For this review, take the finished solid that the model builds, in its own axes (mm). Round coordinates to 2 decimals unless told otherwise and drop trailing zeros. Write each loop counter-clockwise with the first axis right and the second up, starting at its lowest first coordinate (ties: lowest second). Pieces come first, ordered by that corner, then holes. Notation, with made-up numbers: (27, -24.75) - (74, -24.75) arc R14 cw to (74, -20.75) - close; hole circle Ø7 at (83, 89.5). An arc over 180 degrees is marked (long way). One line per item, written item: value. Start each with the question number.
Q1. Add section C-C on z = -33.5. Write out the cut boundary in (x, y), and give its area (3 significant figures).
Q2. Clearance check with flat-ended pins moving along their axes: pin 1 Ø12 at (y, z) = (2.5, -12) entering from -X; pin 2 Ø3.5 at (x, y) = (0, 28.5) entering from +Z; pin 3 Ø7 at (x, y) = (0.5, -31) entering from -Z. State where each tip first meets the part, or that it passes through.
Q3. Add section A-A on z = 0. Write out the cut boundary in (x, y) (3 decimals), and give its area (3 significant figures).
Q4. Add section D-D on y = -36. Write out the cut boundary in (x, z).
Q5. For probe 1 along Y at (x, z) = (-7.9, 0) (3 decimals); probe 2 along Z at (x, y) = (2, 17); probe 3 along Y at (x, z) = (-0.75, 0) (3 decimals), list the stretches that pass through material, from the lowest coordinate up.
Autodesk Inventor part; units mm, degrees
ref_plane "YZ Plane" through (0, 0, 0) normal (1, 0, 0) x (0, 1, 0)
ref_plane "XZ Plane" through (0, 0, 0) normal (0, 1, 0) x (-1, 0, 0)
ref_plane "XY Plane" through (0, 0, 0) normal (0, 0, 1) x (1, 0, 0)
sketch "Sketch1" plane through (0, 0, 0) normal (1, 0, 0) x (0, 1, 0)
  circle A0 centre (0, 0) radius 44
  dimension "d0" = 88
extrude "Extrusion1" add sketch "Sketch1" along normal blind 3.5
sketch "Sketch2" plane through (3.5, 0, 0) normal (1, 0, 0) x (0, 0, -1)
  circle A0 centre (0, 0) radius 45
  dimension "d3" = 90
extrude "Extrusion2" add sketch "Sketch2" along normal blind 1
sketch "Sketch3" plane through (0, 0, 0) normal (-1, 0, 0) x (0, 0, 1)
  circle A0 centre (0, 0) radius 45
  dimension "d6" = 90
extrude "Extrusion3" add sketch "Sketch3" along normal blind 1
sketch "Sketch4" plane through (4.5, 0, 0) normal (1, 0, 0) x (0, 0, -1)
  circle A0 centre (0, 0) radius 41.5
  dimension "d9" = 83
extrude "Extrusion4" cut sketch "Sketch4" against normal blind 6
sketch "Sketch5" plane through (4.5, 0, 0) normal (1, 0, 0) x (0, 0, -1)
  circle A0 centre (0, 0) radius 3.5
  dimension "d12" = 7
extrude "Extrusion5" add sketch "Sketch5" against normal blind 10
sketch "Sketch6" plane through (4.5, 0, 0) normal (1, 0, 0) x (0, 0, -1)
  circle A0 centre (0, 0) radius 45
extrude "Extrusion6" cut sketch "Sketch6" against normal blind 2
sketch "Sketch7" plane through (2.5, 0, 0) normal (1, 0, 0) x (0, 0, -1)
  circle A0 centre (0, 0) radius 3.5
  circle A1 centre (0, 0) radius 41.5
  circle A2 centre (0, 0) radius 45
extrude "Extrusion7" add sketch "Sketch7" along normal blind 1 contours A2
sketch "Sketch8" plane through (2.5, 0, 0) normal (1, 0, 0) x (0, 0, -1)
  circle A0 centre (0, 0) radius 3.5
extrude "Extrusion8" add sketch "Sketch8" along normal blind 1
sketch "Sketch9" plane through (3.5, 0, 0) normal (1, 0, 0) x (0, 0, -1)
  circle A0 centre (0, 0) radius 1.625
  dimension "d21" = 3.25
extrude "Extrusion9" cut sketch "Sketch9" against normal blind 10
sketch "Sketch10" plane through (3.5, 0, 0) normal (1, 0, 0) x (0, 0, -1)
  line L0 (2, 2.1756) -> (-2, 2.1756)
  line L1 (-2, 2.1756) -> (-2, 42.8244)
  line L2 (-2, 42.8244) -> (2, 42.8244)
  line L3 (2, 42.8244) -> (2, 2.1756)
  line L4 (2, 2.1756) -> (-2, 42.8244) construction
  line L5 (-2, 2.1756) -> (2, 42.8244) construction
  point P0 (0, 0)
  point P1 (0, 22.5)
  dimension "d24" = 4
extrude "Extrusion10" add sketch "Sketch10" against normal blind 4.5
pattern_circular "Circular Pattern1" count 4 over 360 about axis through (4.5, 0, 0) along (-1, 0, 0) of "Extrusion10"
fillet "Fillet1" radius 2 5 edges at (-1, 0, 3.5) (-1, -3.5, 0) (-1, 3.5, 0) (-1, -1.0481, -3.3394) (-1, 1.0481, -3.3394)
sketch "Sketch11" plane through (-5.5, 0, 0) normal (-1, 0, 0) x (0, 0, 1)
  circle A0 centre (0, 0) radius 1.625
  circle A1 centre (0, 0) radius 3.5
extrude "Extrusion11" add sketch "Sketch11" along normal blind 2
sketch "Sketch12" plane through (-7.5, 0, 0) normal (-1, 0, 0) x (0, 0, 1)
  circle A0 centre (0, 0) radius 1.625
  circle A1 centre (0, 0) radius 3.5
extrude "Extrusion12" add sketch "Sketch12" along normal blind 1
properties part number "mtv_pushingWheel_2-6"
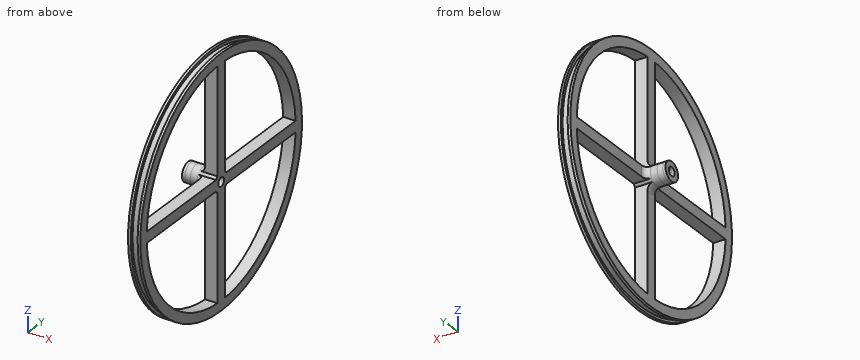
Result set:
1. outline: (-1, -30.05) - (0, -30.05) - (0, -28.53) - (2.5, -28.53) - (2.5, -30.05) - (3.5, -30.05) - (3.5, -24.49) - (-1, -24.49) - close; (-1, -2) - (3.5, -2) - (3.5, 2) - (-1, 2) - close; (-1, 24.49) - (3.5, 24.49) - (3.5, 30.05) - (2.5, 30.05) - (2.5, 28.53) - (0, 28.53) - (0, 30.05) - (-1, 30.05) - close
1. area: 60.4 mm^2
2. pin 1: stops at x = -1
2. pin 2: stops at z = 36.19
2. pin 3: stops at z = -35.59
3. outline: (-8.5, -3.5) - (-3, -3.5) arc R2 cw to (-1, -5.5) - (-1, -45) - (0, -45) - (0, -44) - (2.5, -44) - (2.5, -45) - (3.5, -45) - (3.5, -1.625) - (-8.5, -1.625) - close; (-8.5, 1.625) - (3.5, 1.625) - (3.5, 45) - (2.5, 45) - (2.5, 44) - (0, 44) - (0, 45) - (-1, 45) - (-1, 5.5) arc R2 cw to (-3, 3.5) - (-8.5, 3.5) - close
3. area: 415 mm^2
4. outline: (-1, -27) - (0, -27) - (0, -25.3) - (2.5, -25.3) - (2.5, -27) - (3.5, -27) - (3.5, -20.65) - (-1, -20.65) - close; (-1, -2) - (3.5, -2) - (3.5, 2) - (-1, 2) - close; (-1, 20.65) - (3.5, 20.65) - (3.5, 27) - (2.5, 27) - (2.5, 25.3) - (0, 25.3) - (0, 27) - (-1, 27) - close
5. probe 1: y = -3.5 to -1.625, 1.625 to 3.5
5. probe 2: z = -40.58 to -37.86, -2 to 2, 37.86 to 40.58
5. probe 3: y = -45 to -1.625, 1.625 to 45
